from build123d import *

# Parameters (mm, degrees)
SALIENTE_EXTRUIR1_DEPTH             = 116
CROQUIS2_W                          = 6
CROQUIS2_H                          = 13.55
CORTAR_EXTRUIR1_DEPTH               = 85.315116124
CROQUIS3_W                          = 6
CROQUIS3_H                          = 13.55
CORTAR_EXTRUIR2_DEPTH               = 85.315116124
CORTAR_EXTRUIR3_DEPTH               = 85.315116124
CORTAR_EXTRUIR4_DEPTH               = 85.069267231
DI_METRO_DE_TALADRO_2_5_2_5_1_D     = 2.5
DI_METRO_DE_TALADRO_3_0_3_1_D       = 3
DI_METRO_DE_TALADRO_1_6_1_6_1_D     = 1.6
DI_METRO_DE_TALADRO_4_0_4_1_D       = 4
DI_METRO_DE_TALADRO_4_0_4_1_DEPTH   = 12.9748366
DI_METRO_DE_TALADRO_1_6_1_6_2_D     = 1.6
DI_METRO_DE_TALADRO_1_6_1_6_2_DEPTH = 12.9748366
DI_METRO_DE_TALADRO_4_2_4_2_1_D     = 4.2
REDONDEO1_R                         = 0.6
REDONDEO2_R                         = 1.5
REDONDEO3_R                         = 2
REDONDEO4_R                         = 3
SALIENTE_EXTRUIR2_DEPTH             = 4
SALIENTE_EXTRUIR2_DEPTH_BACK        = 4
CROQUIS18_W                         = 116
CROQUIS18_H                         = 1.5
REDONDEO5_R                         = 4


with BuildPart() as part:
    # Croquis1 → Saliente-Extruir1 (new body)
    with BuildSketch(Plane(origin=(0, 0, -57), x_dir=(-1, 0, 0), z_dir=(0, 0, -1))):
        Polygon((58.4496732, -13.25), (35.5, 0), (-38, 0), (-38, -1.5), (35.098076211, -1.5), (57.6996732, -14.549038106), align=None)
    extrude(amount=-SALIENTE_EXTRUIR1_DEPTH)

    # Croquis2 → Cortar-Extruir1 (cut, through all)
    with BuildSketch(Plane(origin=(0, 0, 0), x_dir=(-1, 0, 0), z_dir=(0, 1, 0))):
        with Locations((-14.07, -18.5)):
            Rectangle(CROQUIS2_W, CROQUIS2_H)
    extrude(amount=-CORTAR_EXTRUIR1_DEPTH, mode=Mode.SUBTRACT)

    # Croquis3 → Cortar-Extruir2 (cut, through all)
    with BuildSketch(Plane(origin=(0, 0, 0), x_dir=(-1, 0, 0), z_dir=(0, 1, 0))):
        with Locations((-14.07, -0.5)):
            Rectangle(CROQUIS3_W, CROQUIS3_H)
    extrude(amount=-CORTAR_EXTRUIR2_DEPTH, mode=Mode.SUBTRACT)

    # Croquis4 → Cortar-Extruir3 (cut, through all)
    with BuildSketch(Plane(origin=(0, 0, 0), x_dir=(-1, 0, 0), z_dir=(0, 1, 0))):
        with BuildLine():
            Line((21, -4), (21, 6))
            ThreePointArc((21, 6), (20, 7), (19, 6))
            Line((19, 6), (19, -4))
            ThreePointArc((19, -4), (20, -5), (21, -4))
        make_face()
    extrude(amount=-CORTAR_EXTRUIR3_DEPTH, mode=Mode.SUBTRACT)

    # Croquis5 → Cortar-Extruir4 (cut, through all)
    with BuildSketch(Plane.XZ.offset(1.5)):
        with BuildLine():
            Line((-24, -7), (-24, 9))
            ThreePointArc((-24, 9), (-25, 10), (-26, 9))
            Line((-26, 9), (-26, -7))
            ThreePointArc((-26, -7), (-25, -8), (-24, -7))
        make_face()
    extrude(amount=-CORTAR_EXTRUIR4_DEPTH, mode=Mode.SUBTRACT)

    # Diámetro de taladro Ø2.5 (2.5)1 (through all)
    with Locations(Plane(origin=(0, -1.5, 0), x_dir=(-1, 0, 0), z_dir=(0, -1, 0))):
        with Locations((-34, -1)):
            Hole(DI_METRO_DE_TALADRO_2_5_2_5_1_D / 2)

    # Diámetro de taladro Ø3.0 (3)1 (through all)
    with Locations(Plane(origin=(0, -1.5, 0), x_dir=(-1, 0, 0), z_dir=(0, -1, 0))):
        with Locations((-15.15, -24), (-31.5, 53.5), (20.5, -55.5), (-31.5, -55.5), (20.5, 53.5)):
            Hole(DI_METRO_DE_TALADRO_3_0_3_1_D / 2)

    # Diámetro de taladro Ø1.6 (1.6)1 (through all)
    with Locations(Plane(origin=(0, -1.5, 0), x_dir=(-1, 0, 0), z_dir=(0, -1, 0))):
        with Locations((22.75, -15), (22.75, 13)):
            Hole(DI_METRO_DE_TALADRO_1_6_1_6_1_D / 2)

    # Diámetro de taladro Ø4.0 (4)1
    with Locations(Plane(origin=(-8.125, 14.072912811, 0), x_dir=(-0.8660254037844288, -0.5000000000000172, 0), z_dir=(0.5000000000000172, -0.8660254037844288, 0))):
        with Locations((44.743901834, -1)):
            Hole(DI_METRO_DE_TALADRO_4_0_4_1_D / 2, depth=DI_METRO_DE_TALADRO_4_0_4_1_DEPTH)

    # Diámetro de taladro Ø1.6 (1.6)2
    with Locations(Plane(origin=(-8.125, 14.072912811, 0), x_dir=(-0.8660254037844288, -0.5000000000000172, 0), z_dir=(0.5000000000000172, -0.8660254037844288, 0))):
        with Locations((44.743901834, -19), (44.743901834, 17)):
            Hole(DI_METRO_DE_TALADRO_1_6_1_6_2_D / 2, depth=DI_METRO_DE_TALADRO_1_6_1_6_2_DEPTH)

    # Diámetro de taladro Ø4.2 (4.2)1 (through all)
    with Locations(Plane(origin=(0, -1.5, 0), x_dir=(-1, 0, 0), z_dir=(0, -1, 0))):
        with Locations((31, -53), (31, 51), (-22, -53), (-22, 51), (-15.15, -15)):
            Hole(DI_METRO_DE_TALADRO_4_2_4_2_1_D / 2)

    # Redondeo1
    redondeo1_edges = [part.edges().sort_by_distance(p)[0] for p in [
        (17.07, -0.75, -25.275),
        (17.07, -0.75, -11.725),
        (11.07, -0.75, -11.725),
        (11.07, -0.75, -25.275),
        (11.07, -0.75, -7.275),
        (17.07, -0.75, -7.275),
        (17.07, -0.75, 6.275),
        (11.07, -0.75, 6.275),
    ]]
    fillet(redondeo1_edges, radius=REDONDEO1_R)

    # Redondeo2
    redondeo2_edges = [part.edges().sort_by_distance(p)[0] for p in [
        (-35.098076211, -1.5, 1),
    ]]
    fillet(redondeo2_edges, radius=REDONDEO2_R)

    # Redondeo3
    redondeo3_edges = [part.edges().sort_by_distance(p)[0] for p in [
        (38, -0.75, 59),
        (-58.0746732, -13.899519053, 59),
        (38, -0.75, -57),
        (-58.0746732, -13.899519053, -57),
    ]]
    fillet(redondeo3_edges, radius=REDONDEO3_R)

    # Redondeo4
    redondeo4_edges = [part.edges().sort_by_distance(p)[0] for p in [
        (-35.5, 0, 1),
    ]]
    fillet(redondeo4_edges, radius=REDONDEO4_R)

    # Croquis18 → Saliente-Extruir2 (add, two sides: drawn at the far end of the back side and taken through both)
    with BuildSketch(Plane(origin=(38, 0, 0), x_dir=(0, 0, -1), z_dir=(1, 0, 0)).offset(-SALIENTE_EXTRUIR2_DEPTH_BACK)):
        with Locations((-1, -0.75)):
            Rectangle(CROQUIS18_W, CROQUIS18_H)
    extrude(amount=SALIENTE_EXTRUIR2_DEPTH + SALIENTE_EXTRUIR2_DEPTH_BACK)

    # Redondeo5
    redondeo5_edges = [part.edges().sort_by_distance(p)[0] for p in [
        (42, -0.75, 59),
        (42, -0.75, -57),
    ]]
    fillet(redondeo5_edges, radius=REDONDEO5_R)


solid = part.part
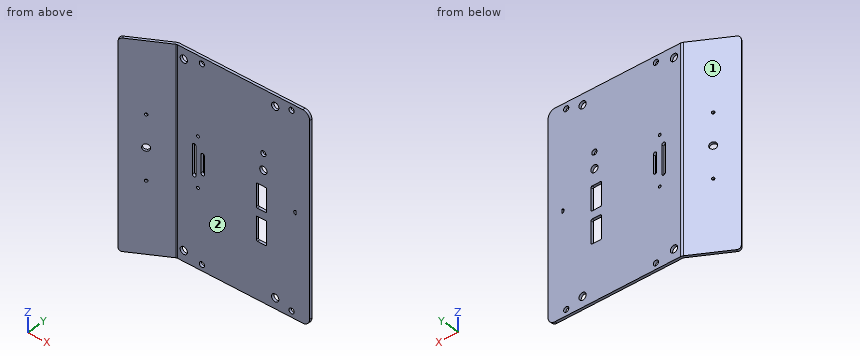
Input: part model. Units: mm. Frame: model coordinates. Face numbers are marked on the shaded views. A direction names the side the tool comes from. Coordinates: 2 decimals unless noted, no trailing zeros. Loops run counter-clockwise (first coordinate to the right, second up) from the corner with the lowest first, then second, coordinate; pieces in that order, holes last. Notation, with made-up numbers: (72.25, -39) -> (84.25, -39) arc R10 ccw to (84.25, -22) -> close; hole circle Ø11 at (-6.5, -0.75). An arc over 180 degrees is marked (long way). Write item = value, one per line. Start each with the question number.
Item 1: First-contact query: P1, Ø1.3, axis at x = -22.75, z = -13, coming from the -Y side; P2, Ø1.6, axis at y = -1, z = -2.5, coming from the -X side; P3, Ø5, axis at x = 15.15, z = 24, coming from the -Y side; P4, Ø1, axis at y = -8.5, z = -31.5, coming from the -X side. Flat tips, straight axial feed; report the tip coordinate or a pass-through.
Item 2: Material intervals for line 1 (Z direction, x = 22, y = -1.05); line 2 (Z direction, x = 31.5, y = -0.55); line 3 (Z direction, x = 15.15, y = -0.6) (3 decimals), sorted ascending.
Item 3: Cut plane C-C, the plane y = -3.25. Return loops of the section in (x, z).
Item 4: Cut plane A-A, the plane x = 31.5. Return loops of the section in (y, z).
Item 5: Cut plane D-D, the plane x = -1. Return loops of the section in (y, z), plus the area to 3 significant figures.
Item 6: Reachability of the marked faces 1 and 2 from +Z, -Z, +X, -X, +Y, -Y: full face, straight path, thin tool, end or side. Return the list, or none.
Item 7: Cut plane B-B, the plane z = 42. Return loops of the section in (x, y).
Ans:
q1.P1 = through
q1.P2 = -38.62
q1.P3 = -1.5
q1.P4 = -51.09
q2.line_1 = -57 to -53.1, -48.9 to 50.9, 55.1 to 59
q2.line_2 = -57 to -55, -52 to 54, 57 to 59
q2.line_3 = -57 to -25.275, -11.725 to -7.275, 6.275 to 12.9, 17.1 to 22.5, 25.5 to 59
q3.outline = (-41.13, -57) -> (-38.13, -57) -> (-38.13, 59) -> (-41.13, 59) -> close
q4.outline = (-1.5, -57) -> (0, -57) -> (0, -55) -> (-1.5, -55) -> close; (-1.5, -52) -> (0, -52) -> (0, 54) -> (-1.5, 54) -> close; (-1.5, 57) -> (0, 57) -> (0, 59) -> (-1.5, 59) -> close
q5.outline = (-1.5, -57) -> (0, -57) -> (0, 59) -> (-1.5, 59) -> close
q5.area = 174 mm²
q6.face_1 = +Z, -Z, -X, +Y
q6.face_2 = +Z, -Z, +X, -Y
q7.outline = (-58.45, -13.25) -> (-57.7, -14.55) -> (-35.45, -1.7) arc R1.5 cw to (-34.7, -1.5) -> (42, -1.5) -> (42, 0) -> (-34.7, 0) arc R3 ccw to (-36.2, -0.4) -> close
